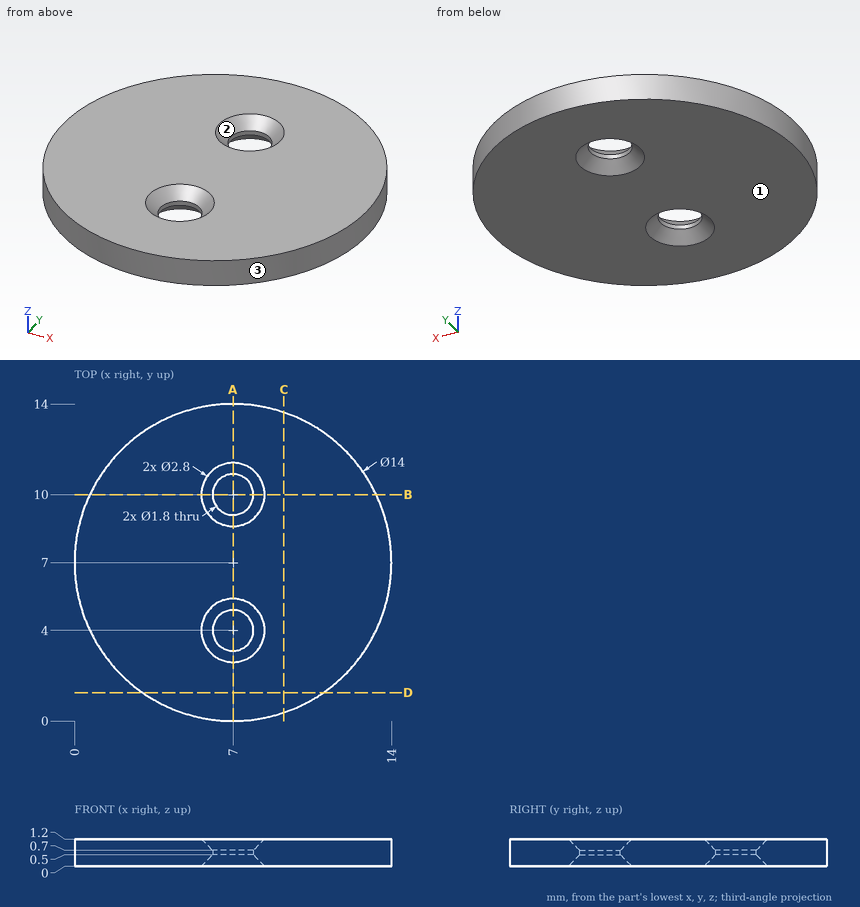
Design review of the part shown in the three views and the two pictorial views. Dimensions are in mm from the part's minimum x, y and z. Coordinates: 2 decimals unless noted, no trailing zeros. Order: outer loops, then holes, each group sorted by start corner. A loop starts at its lowest first (then second) coordinate and runs counter-clockwise, first axis right, second up. Notation, with made-up numbers: (38, -25.75) -> (65, -25.75) arc R22 ccw to (65, 9.25) -> close; hole circle Ø2 at (2, 70.5). An arc over 180 degrees is marked (long way). Use one line per item in the form item = value. Start each with the question number.
(1) Insertion check: pin 1 (2 mm diameter, centred on x = 7, y = 10, fed in from -Z); pin 2 (3 mm diameter, centred on x = 7, y = 4, fed in from +Z). Each pin has a flat end and moves straight along its axis. Give the tip position at first contact, or say it passes through.
(2) Add section B-B on y = 10. State the section outline as (x, z) points.
(3) The part is to be moulded in two halves that separate along X. For the marked faces 1, 2 and 3, say which applies: +X half, -X half, draft (parallel to the pull), parting line (faces both ways), or undercut.
(4) For probe 1 along Y at (x, z) = (7, 0.55); probe 2 along X at (y, z) = (4, 0.6); probe 3 along X at (y, z) = (3.25, 0.45), list the stretches that pass through material, from the lowest coordinate up.
(5) Add section D-D on y = 1.25. State the section outline as (x, z) points.
(6) Add section A-A on x = 7. State the section outline as (y, z) points, plus the area to 3 significant figures.
(7) Add section C-C on x = 9.25. State the section outline as (y, z) points.
Answer block:
q1.pin_1 = 0.4
q1.pin_2 = 1.2
q2.outline = (0.68, 0) -> (5.6, 0) -> (6.1, 0.5) -> (6.1, 0.7) -> (5.6, 1.2) -> (0.68, 1.2) -> close; (7.9, 0.5) -> (8.4, 0) -> (13.32, 0) -> (13.32, 1.2) -> (8.4, 1.2) -> (7.9, 0.7) -> close
q3.face_1 = draft
q3.face_2 = undercut
q3.face_3 = parting line
q4.probe_1 = 0 to 3.1, 4.9 to 9.1, 10.9 to 14
q4.probe_2 = 0.68 to 6.1, 7.9 to 13.32
q4.probe_3 = 1.09 to 6.42, 7.58 to 12.91
q5.outline = (3.01, 0) -> (10.99, 0) -> (10.99, 1.2) -> (3.01, 1.2) -> close
q6.outline = (0, 0) -> (2.6, 0) -> (3.1, 0.5) -> (3.1, 0.7) -> (2.6, 1.2) -> (0, 1.2) -> close; (4.9, 0.5) -> (5.4, 0) -> (8.6, 0) -> (9.1, 0.5) -> (9.1, 0.7) -> (8.6, 1.2) -> (5.4, 1.2) -> (4.9, 0.7) -> close; (10.9, 0.5) -> (11.4, 0) -> (14, 0) -> (14, 1.2) -> (11.4, 1.2) -> (10.9, 0.7) -> close
q6.area = 11.5 mm²
q7.outline = (0.37, 0) -> (13.63, 0) -> (13.63, 1.2) -> (0.37, 1.2) -> close
